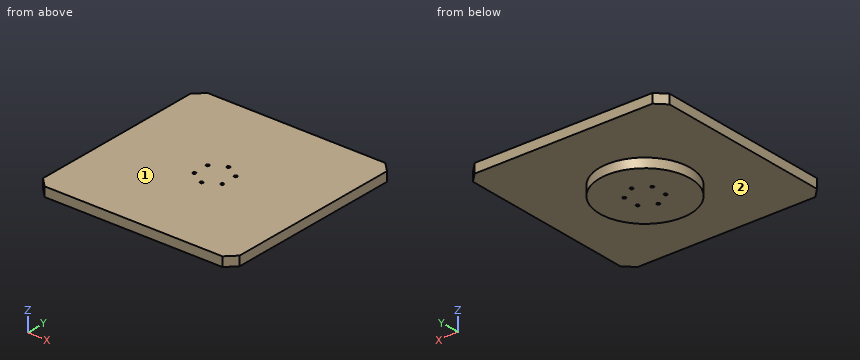
```python
from build123d import *

# Parameters (mm, degrees)
SKETCH_1_W               = 150
SKETCH_1_H               = 150
EXTRUDE_1_DEPTH          = 30
SKETCH_2_R               = 48.25
EXTRUDE_2_DEPTH          = 10
SKETCH_3_R               = 1.65
EXTRUDE_3_DEPTH          = 8.3
SKETCH_4_W               = 150
SKETCH_4_H               = 30
EXTRUDE_4_DEPTH          = 30
SKETCH_5_W               = 30
SKETCH_5_H               = 180
EXTRUDE_5_DEPTH          = 30
SKETCH_6_W               = 180
SKETCH_6_H               = 30
EXTRUDE_6_DEPTH          = 30
SKETCH_7_W               = 30
SKETCH_7_H               = 210
EXTRUDE_7_DEPTH          = 30
CHAMFER_1_SIZE           = 10
CUT_EXTRUDE_1_DEPTH      = 154.785564992
CUT_EXTRUDE_1_DEPTH_BACK = 154.785564992
SKETCH_8_R               = 1.65
CUT_EXTRUDE_START        = -15
SKETCH_9_R               = 48.25
CUT_EXTRUDE_2_DEPTH      = 15
SKETCH_10_R              = 48.25
CUT_EXTRUDE_3_DEPTH      = 15
CUT_EXTRUDE_START_2      = -5
SKETCH_11_R              = 48.25
CUT_EXTRUDE_4_DEPTH      = 5
SKETCH_12_R              = 48.25
CUT_EXTRUDE_5_DEPTH      = 5


with BuildPart() as part:
    # 草图1 → 凸台-拉伸1 (new body)
    with BuildSketch(Plane.XY):
        Rectangle(SKETCH_1_W, SKETCH_1_H)
    extrude(amount=EXTRUDE_1_DEPTH)

    # 草图2 → 凸台-拉伸2 (add)
    with BuildSketch(Plane(origin=(0, 0, 0), x_dir=(-1, 0, 0), z_dir=(0, 0, -1))):
        Circle(SKETCH_2_R)
    extrude(amount=EXTRUDE_2_DEPTH)

    # 草图3 → 凸台-拉伸3 (add)
    with BuildSketch(Plane(origin=(0, 0, -10), x_dir=(-1, 0, 0), z_dir=(0, 0, -1))):
        with Locations(Location((0, 17.25, 0), (0, 0, 180))):
            Circle(SKETCH_3_R)
        with Locations(Location((14.938938215, 8.625, 0), (0, 0, 180))):
            Circle(SKETCH_3_R)
        with Locations(Location((14.938938215, -8.625, 0), (0, 0, 180))):
            Circle(SKETCH_3_R)
        with Locations(Location((0, -17.25, 0), (0, 0, 180))):
            Circle(SKETCH_3_R)
        with Locations(Location((-14.938938215, -8.625, 0), (0, 0, 180))):
            Circle(SKETCH_3_R)
        with Locations(Location((-14.938938215, 8.625, 0), (0, 0, 180))):
            Circle(SKETCH_3_R)
    extrude(amount=EXTRUDE_3_DEPTH)

    # 草图4 → 凸台-拉伸4 (add)
    with BuildSketch(Plane(origin=(0, 75, 0), x_dir=(1, 0, 0), z_dir=(0, 1, 0))):
        with Locations((0, -15)):
            Rectangle(SKETCH_4_W, SKETCH_4_H)
    extrude(amount=EXTRUDE_4_DEPTH)

    # 草图5 → 凸台-拉伸5 (add)
    with BuildSketch(Plane.ZY.offset(75)):
        with Locations((15, 15)):
            Rectangle(SKETCH_5_W, SKETCH_5_H)
    extrude(amount=EXTRUDE_5_DEPTH)

    # 草图6 → 凸台-拉伸6 (add)
    with BuildSketch(Plane.XZ.offset(75)):
        with Locations((-15, 15)):
            Rectangle(SKETCH_6_W, SKETCH_6_H)
    extrude(amount=EXTRUDE_6_DEPTH)

    # 草图7 → 凸台-拉伸7 (add)
    with BuildSketch(Plane(origin=(75, 0, 0), x_dir=(0, 0, -1), z_dir=(1, 0, 0))):
        with Locations((-15, 0)):
            Rectangle(SKETCH_7_W, SKETCH_7_H)
    extrude(amount=EXTRUDE_7_DEPTH)

    # 倒角1
    chamfer_1_edges = [part.edges().sort_by_distance(p)[0] for p in [
        (-105, 105, 15),
        (-105, -105, 15),
        (105, -105, 15),
        (105, 105, 15),
    ]]
    chamfer(chamfer_1_edges, length=CHAMFER_1_SIZE)

    # 草图8 → 切除-拉伸1 (cut, two sides: drawn at the far end of the back side and taken through both)
    with BuildSketch(Plane(origin=(0, 0, -10), x_dir=(-1, 0, 0), z_dir=(0, 0, -1)).offset(-CUT_EXTRUDE_1_DEPTH_BACK)):
        with Locations((-14.938938215, -8.625)):
            Circle(SKETCH_8_R)
        with Locations((0, -17.25)):
            Circle(SKETCH_8_R)
        with Locations((14.938938215, -8.625)):
            Circle(SKETCH_8_R)
        with Locations((14.938938215, 8.625)):
            Circle(SKETCH_8_R)
        with Locations((0, 17.25)):
            Circle(SKETCH_8_R)
        with Locations((-14.938938215, 8.625)):
            Circle(SKETCH_8_R)
    extrude(amount=CUT_EXTRUDE_1_DEPTH + CUT_EXTRUDE_1_DEPTH_BACK, mode=Mode.SUBTRACT)

    # 草图9 → 切除-拉伸2 (cut)
    with BuildSketch(Plane(origin=(0, 0, 0), x_dir=(-1, 0, 0), z_dir=(0, 0, -1)).offset(CUT_EXTRUDE_START)):
        Polygon((-95, -105), (95, -105), (105, -95), (105, 95), (95, 105), (-95, 105), (-105, 95), (-105, -95), align=None)
        Circle(SKETCH_9_R, mode=Mode.SUBTRACT)
    extrude(amount=CUT_EXTRUDE_2_DEPTH, mode=Mode.SUBTRACT)

    # 草图10 → 切除-拉伸3 (cut)
    with BuildSketch(Plane(origin=(0, 0, -10), x_dir=(-1, 0, 0), z_dir=(0, 0, -1)).offset(CUT_EXTRUDE_START)):
        Circle(SKETCH_10_R)
    extrude(amount=CUT_EXTRUDE_3_DEPTH, mode=Mode.SUBTRACT)

    # 草图11 → 切除-拉伸4 (cut)
    with BuildSketch(Plane(origin=(0, 0, 5), x_dir=(-1, 0, 0), z_dir=(0, 0, -1)).offset(CUT_EXTRUDE_START_2)):
        Circle(SKETCH_11_R)
    extrude(amount=CUT_EXTRUDE_4_DEPTH, mode=Mode.SUBTRACT)

    # 草图12 → 切除-拉伸5 (cut)
    with BuildSketch(Plane(origin=(0, 0, 15), x_dir=(-1, 0, 0), z_dir=(0, 0, -1)).offset(CUT_EXTRUDE_START_2)):
        Polygon((-105, -95), (-95, -105), (95, -105), (105, -95), (105, 95), (95, 105), (-95, 105), (-105, 95), align=None)
        Circle(SKETCH_12_R, mode=Mode.SUBTRACT)
    extrude(amount=CUT_EXTRUDE_5_DEPTH, mode=Mode.SUBTRACT)


solid = part.part
```
Could you check a few things on this model? Use its own coordinates, in mm. Face numbers are marked on the shaded views. A direction names the side the tool comes from. Round coordinates to 2 decimals unless told otherwise and drop trailing zeros. Loops run counter-clockwise (first coordinate to the right, second up) from the corner with the lowest first, then second, coordinate; pieces in that order, holes last. Notation, with made-up numbers: M 66,-8.75 L 122,-8.75 A15 cw 122,10.25 Z; hole C 48.5,2 d1. An arc over 180 degrees is marked long. Put each result on its own line as item: value.
Q1. Imagine slicing it at C-C (y = -54). Write out the boundary of the cut face in (x, z), then the cut area to 3 significant figures.
Check result:
outline: M -105,20 L 105,20 L 105,30 L -105,30 Z
area: 2,100 mm2
Q2. For pin 1 (8 mm diameter, centred on y = 34.5, z = 16.5, fed in from -X); pin 2 (4 mm diameter, centred on x = 15, z = 15.5, fed in from +Y); pin 3 (5 mm diameter, centred on y = 17, z = 16.5, fed in from -X), each with a flat end and sliding along its axis, tell me the tip position at first contact or that it passes through.
Check result:
pin 1: x = -105
pin 2: y = 46.47
pin 3: x = -46.02
Q3. Imagine slicing it at A-A (y = 0). Write out the boundary of the cut face in (x, z).
Check result:
outline: M -105,20 L -48.25,20 L -48.25,10 L 48.25,10 L 48.25,20 L 105,20 L 105,30 L -105,30 Z
Q4. On a 3-axis mill with a long thin cutter (end or side, diameter ignored), from which of +Z, -Z, +X, -X, +Y, -Y can I reach the whole of each face in a straight line? I mean the marked faces 1 and 2. Say none if no direction works.
Check result:
face 1: +Z, +X, -X, +Y, -Y
face 2: -Z
Q5. I need wall thicknesses on probe 1 along Y at (x, z) = (0, 18); probe 2 along Y at (x, z) = (0, 22.75); probe 3 along X at (y, z) = (-9, 15.5). Which ranges of each line are inside material? Lowest first, please.
Check result:
probe 1: -48.25 to -18.9, -15.6 to 15.6, 18.9 to 48.25
probe 2: -105 to -18.9, -15.6 to 15.6, 18.9 to 105
probe 3: -47.4 to -16.55, -13.33 to 13.33, 16.55 to 47.4
Q6. Imagine slicing it at B-B (x = 6.5). Write out the boundary of the cut face in (y, z).
Check result:
outline: M -105,20 L -47.81,20 L -47.81,10 L 47.81,10 L 47.81,20 L 105,20 L 105,30 L -105,30 Z
